CAD build for the part. Positions are in the model's coordinates, mm. A direction names the side the tool comes from. Coordinates: 2 decimals unless noted, no trailing zeros. Loops run counter-clockwise (first coordinate to the right, second up) from the corner with the lowest first, then second, coordinate; pieces in that order, holes last. Notation, with made-up numbers: (50.25, -26.75) -> (90.25, -26.75) arc R14 ccw to (90.25, -4.75) -> close; hole circle Ø10 at (18, 80). An arc over 180 degrees is marked (long way). Write each question's results on one line, items separated by ' | '.
```python
from build123d import *

# Parameters (mm, degrees)
F2_SIZE  = 0.75
F3_SIZE2 = 3
F3_SIZE  = 5.1961524227
F5_D     = 5.4102
F5_DEPTH = 21.721
F5_TIP   = 1.6253880605


with BuildPart() as f1:
    # F0 (on Front) → F1 (revolve)
    with BuildSketch(Plane.XZ):
        Polygon((-32, 0), (0, 0), (0, 70.85), (-9.5, 70.85), (-9.5, 7.35), (-39.5, 7.35), (-39.5, 1), (-32, 1), align=None)
    revolve(axis=Axis((0, 0, 35.425), (0, 0, -1)))

    # F2
    f2_edges = [f1.edges().sort_by_distance(p)[0] for p in [
        (9.5, 0, 70.85),
        (9.5, 0, 7.35),
    ]]
    chamfer(f2_edges, length=F2_SIZE)

    # F3
    f3_edges = [f1.edges().sort_by_distance(p)[0] for p in [
        (39.5, 0, 7.35),
    ]]
    f3_side = f1.faces().sort_by_distance((11.367229, 0, 7.35))[0]
    chamfer(f3_edges, length=F3_SIZE, length2=F3_SIZE2, reference=f3_side)

    # F5
    with Locations(Plane(origin=(0, 0, 0), x_dir=(1, 0, 0), z_dir=(0, 0, -1))):
        with Locations((0, 0)):
            Hole(F5_D / 2, depth=F5_DEPTH)
            with Locations((0, 0, -(F5_DEPTH + F5_TIP / 2))):  # 118° drill point
                Cone(0, F5_D / 2, F5_TIP, mode=Mode.SUBTRACT)


solid = f1.part
```
Q1. Which spindle directions (+Z, -Z, +X, -X, +Y, -Y) get a long thin tool onto all of the face, cutting with end or side? Do faces 1 (the flat face through (3.11, -32, 1)), 2 (the flat face through (0, 0, 70.85)), 3 (the cylindrical face through (-4.38, -8.43, 38.67)). Say none if no direction does.
Results are:
face 1: -Z | face 2: +Z, +X, -X, +Y, -Y | face 3: +Z
Q2. Drop flat-ended pins along their axis: pin 1 (3 mm diameter, centred on y = 7, z = 56.5, fed in from -X); pin 2 (1.5 mm diameter, centred on x = -23.5, y = -18.5, fed in from +Z); pin 3 (1 mm diameter, centred on y = 4.5, z = 34, fed in from -X). Give the stop position or say it passes through.
Results are:
pin 1: x = -7.75 | pin 2: z = 7.35 | pin 3: x = -8.62
Q3. Pull direction Y, two halves, no side cores. Call faces 4 (the conical face through (7.51, -33.81, 7.16)), 5 (the flat face through (0, -7, 0)), 6 (the conical face through (-0.102, 0.459, 23.064)): +Y half, -Y half, draft (parallel to the pull), parting line (faces both ways), or undercut.
Results are:
face 4: parting line | face 5: draft | face 6: undercut
Q4. Wall check: L1, parallel to Y at x = 0, z = 11.5; L2, parallel to Z at x = 17, y = -8; L3, parallel to Y at x = 0, z = 7. Give the ranges that are in metal, low to high. Write a range as from..to.
Results are:
L1: -9.5..-2.71, 2.71..9.5 | L2: 0..7.35 | L3: -34.91..-2.71, 2.71..34.91
Q5. Cut at A-A on z = 50. Write the cut outline in (x, y), and give its area (3 significant figures).
Results are:
outline: circle Ø19 at (0, 0) | area: 284 mm^2
